Here's how the part is built. I have some questions about the finished solid (model axes, mm). Face numbers are marked on the shaded views. A direction names the side the tool comes from. Round coordinates to 2 decimals unless told otherwise and drop trailing zeros. Loops run counter-clockwise (first coordinate to the right, second up) from the corner with the lowest first, then second, coordinate; pieces in that order, holes last. Notation, with made-up numbers: M 5.25,41.5 L 32.25,41.5 A19 cw 32.25,52.5 Z; hole C 60,33 d9. An arc over 180 degrees is marked long. Use a Markdown table: item, result.
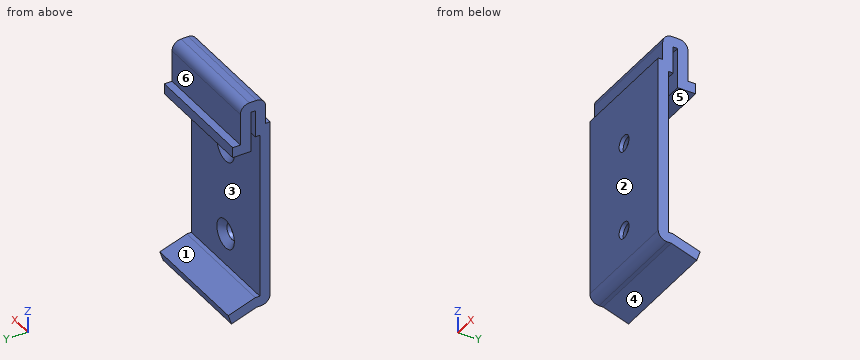
from build123d import *

# Parameters (mm, degrees)
EXTRUDE_1_DEPTH          = 5
FILLET_1_R               = 2
EXTRUDE_3_DEPTH          = 15
HOLE_WIZARD_1_AT_2_COUNT = 2
HOLE_WIZARD_1_AT_2_PITCH = 20


with BuildPart() as part:
    # 草图1 → 凸台-拉伸1 (new, symmetric)
    with BuildSketch(Plane(origin=(0, 0, 0), x_dir=(0, 0, -1), z_dir=(1, 0, 0))):
        Polygon((0, 4), (0, 0), (-9, 0), (-9, -1), (-3, -1), (-3, -2), (34, -2), (34, -1), (36, 5), (38.181971586, 4.272676138), (36.3, -1.373238618), (36.3, -4.3), (-5.3, -4.3), (-5.3, -3.3), (-11.3, -3.3), (-11.3, 2.3), (-2.3, 2.3), (-2.3, 4), align=None)
    extrude(amount=EXTRUDE_1_DEPTH, both=True)

    # 圆角1
    fillet_1_edges = [part.edges().sort_by_distance(p)[0] for p in [
        (0, -4.3, -36.3),
        (0, -3.3, 11.3),
        (0, 2.3, 11.3),
    ]]
    fillet(fillet_1_edges, radius=FILLET_1_R)

    # 草图7 → 凸台-拉伸3 (add)
    with BuildSketch(Plane(origin=(5, 0, 0), x_dir=(0, 0, -1), z_dir=(1, 0, 0))):
        with BuildLine():
            Line((-5.3, -4.3), (34.3, -4.3))
            ThreePointArc((34.3, -4.3), (35.714213562, -3.714213562), (36.3, -2.3))
            Line((36.3, -2.3), (36.3, -1.373238618))
            Line((36.3, -1.373238618), (38.181971586, 4.272676138))
            Line((38.181971586, 4.272676138), (36, 5))
            Line((36, 5), (34, -1))
            Line((34, -1), (34, -2))
            Line((34, -2), (-3, -2))
            Line((-3, -2), (-3, -1))
            Line((-3, -1), (-9, -1))
            Line((-9, -1), (-9, 0))
            Line((-9, 0), (0, 0))
            Line((0, 0), (0, 4))
            Line((0, 4), (-2.3, 4))
            Line((-2.3, 4), (-2.3, 2.3))
            Line((-2.3, 2.3), (-9.3, 2.3))
            ThreePointArc((-9.3, 2.3), (-10.714213562, 1.714213562), (-11.3, 0.3))
            Line((-11.3, 0.3), (-11.3, -1.3))
            ThreePointArc((-11.3, -1.3), (-10.714213562, -2.714213562), (-9.3, -3.3))
            Line((-9.3, -3.3), (-5.3, -3.3))
            Line((-5.3, -3.3), (-5.3, -4.3))
        make_face()
    extrude(amount=EXTRUDE_3_DEPTH)

    # 草图3 → 打孔尺寸开槽半沉头螺钉的类型1 (revolve, cut)
    with BuildSketch(Plane(origin=(7.5, -2, -27), x_dir=(0, 0, 1), z_dir=(1, 0, 0))):
        Polygon((0, 0), (0, 2.3), (1.8, 2.3), (1.8, 1.4), (3.2, 0), align=None)
    hole_wizard_1 = revolve(axis=Axis((7.5, 4.35, -27), (0, -1, 0)), mode=Mode.SUBTRACT)

    # 打孔尺寸开槽半沉头螺钉的类型1 at 2: 打孔尺寸开槽半沉头螺钉的类型1 ×2
    with Locations(*[(0, 0, i * HOLE_WIZARD_1_AT_2_PITCH) for i in range(1, HOLE_WIZARD_1_AT_2_COUNT)]):
        add(hole_wizard_1, mode=Mode.SUBTRACT)


solid = part.part
1. I need wall thicknesses on probe 1 along X at (y, z) = (-3.7, -7); probe 2 along Z at (x, y) = (7.5, -3.9); probe 3 along Y at (x, z) = (4.75, -17). Which ranges of each line are inside material? Lowest first, please. Write a range as from..to.
Answer sheet:
| item | result |
|---|---|
| probe 1 | -5..5.7, 9.3..20 |
| probe 2 | -35.5..-28.8, -25.2..-8.8, -5.2..5.3 |
| probe 3 | -4.3..-2 |
2. We'd pull the mould along Z, two halves only. Please class the marked faces 3, 4, 5 and 6: +Z half, -Z half, draft (parallel to the pull), parting line (faces both ways), or undercut.
Answer sheet:
| item | result |
|---|---|
| face 3 | undercut |
| face 4 | -Z half |
| face 5 | undercut |
| face 6 | draft |
3. Imagine slicing it at D-D, the plane z = 1. Write out the boundary of the cut face in (x, y), then the cut area to 4 significant figures.
Answer sheet:
| item | result |
|---|---|
| outline | M -5,-4.3 L 20,-4.3 L 20,-2 L -5,-2 Z; M -5,0 L 20,0 L 20,4 L -5,4 Z |
| area | 157.5 mm2 |
4. For pin 1 Ø3.5 at (x, z) = (9.5, 6.5) entering from +Y; pin 2 Ø3 at (x, y) = (12, 1.5) entering from -Z; pin 3 Ø3 at (x, z) = (-1, -32) entering from +Y, each with a flat end and sliding along its axis, tell me the tip position at first contact or that it passes through.
Answer sheet:
| item | result |
|---|---|
| pin 1 | y = 2.3 |
| pin 2 | z = -37.76 |
| pin 3 | y = -2 |
5. Imagine slicing it at A-A, the plane z = -7. Write out the boundary of the cut face in (x, y).
Answer sheet:
| item | result |
|---|---|
| outline | M -5,-4.3 L 5.7,-4.3 L 5.7,-3.4 L 4.3,-2 L -5,-2 Z; M 9.3,-4.3 L 20,-4.3 L 20,-2 L 10.7,-2 L 9.3,-3.4 Z |
6. Which directions (+Z, -Z, +X, -X, +Y, -Y) give clear straight access to the entire face, cutting with the end or side of a thin tool? Please do the marked faces 1 and 2.
Answer sheet:
| item | result |
|---|---|
| face 1 | +X, -X, +Y |
| face 2 | +Z, -Z, +X, -X, -Y |
7. Imagine slicing it at B-B, the plane x = 7.5. State how many separate pieces and enclosed holes the cut face has, then the cut area to 3 significant figures.
Answer sheet:
| item | result |
|---|---|
| separate pieces | 3 |
| enclosed holes | 0 |
| area | 137 mm2 |
8. Imagine slicing it at C-C, the plane y = 1. Write out the boundary of the cut face in (x, z).
Answer sheet:
| item | result |
|---|---|
| outline | M -5,-37.09 L 20,-37.09 L 20,-34.67 L -5,-34.67 Z; M -5,0 L 20,0 L 20,11.17 L -5,11.17 Z |
